from build123d import *

# Parameters (mm, degrees)
SKETCH1_R           = 2.1
BOSS_EXTRUDE1_DEPTH = 154
FILLET1_R           = 0.5


with BuildPart() as part:
    # Sketch1 → Boss-Extrude1 (new body)
    with BuildSketch(Plane.XY):
        Polygon((-20, -10), (-15.5, -10), (-15.1, -10), (-13.1, -8), (-15.5, -8), (-15.5, -6.560660172), (-12.539339828, -3.6), (-7.460660172, -3.6), (-4.5, -6.560660172), (-4.5, -8), (-6.9, -8), (-4.9, -10), (5.313777138, -10), (7.313777138, -8), (4.5, -8), (4.5, -6.560660172), (7.460660172, -3.6), (12.539339828, -3.6), (15.5, -6.560660172), (15.5, -8), (13.513777138, -8), (15.1, -10), (15.5, -10), (20, -10), (20, -5.5), (20, -5.1), (18, -3.1), (18, -5.5), (16.560660172, -5.5), (13.6, -2.539339828), (13.6, 2.539339828), (16.560660172, 5.5), (18, 5.5), (18, 3.1), (20, 5.1), (20, 5.5), (20, 10), (15.5, 10), (15.1, 10), (13.1, 8), (15.5, 8), (15.5, 6.560660172), (12.539339828, 3.6), (7.460660172, 3.6), (4.5, 6.560660172), (4.5, 8), (7.313777138, 8), (5.313777138, 10), (-4.9, 10), (-6.9, 8), (-4.5, 8), (-4.5, 6.560660172), (-7.460660172, 3.6), (-12.539339828, 3.6), (-15.5, 6.560660172), (-15.5, 8), (-13.1, 8), (-15.1, 10), (-15.5, 10), (-20, 10), (-20, 5.5), (-20, 5.1), (-18, 3.1), (-18, 5.5), (-16.560660172, 5.5), (-13.6, 2.539339828), (-13.6, -2.539339828), (-16.560660172, -5.5), (-18, -5.5), (-18, -3.1), (-20, -5.1), (-20, -5.5), align=None)
        with Locations((-10, 0)):
            Circle(SKETCH1_R, mode=Mode.SUBTRACT)
        with Locations((10, 0)):
            Circle(SKETCH1_R, mode=Mode.SUBTRACT)
        Polygon((3, -5.939339828), (3, -8), (-3, -8), (-3, -5.939339828), (-6.4, -2.539339828), (-6.4, 2.539339828), (-3, 5.939339828), (-3, 8), (3, 8), (3, 5.939339828), (6.4, 2.539339828), (6.4, -2.539339828), align=None, mode=Mode.SUBTRACT)
    extrude(amount=BOSS_EXTRUDE1_DEPTH)

    # Fillet1
    fillet1_edges = [part.edges().sort_by_distance(p)[0] for p in [
        (-20, 10, 77),
        (20, 10, 77),
        (20, -10, 77),
        (-20, -10, 77),
    ]]
    fillet(fillet1_edges, radius=FILLET1_R)


solid = part.part
CAD build for the part. Positions are in the model's coordinates, mm. A direction names the side the tool comes from. Round coordinates to 2 decimals unless told otherwise and drop trailing zeros. Order: outer loops, then holes, each group sorted by start corner. A loop starts at its lowest first (then second) coordinate and runs counter-clockwise, first axis right, second up. Notation, with made-up numbers: M 67.25,85.25 L 83.25,85.25 A23 ccw 83.25,101.25 Z; hole C 65,-22 d8. An arc over 180 degrees is marked long. Use one line per item in the form item = value.
Q1. Saw through at D-D on z = 13. State how many separate pieces and enclosed holes the cut face has, then the cut area to 3 significant figures.
Recorded:
separate_pieces = 1
enclosed_holes = 3
area = 283 mm^2
Q2. Saw through at B-B on y = 0. Give the cut face in (x, z), then the cut area to 3 significant figures.
Recorded:
outline = M -13.6,0 L -12.1,0 L -12.1,154 L -13.6,154 Z; M -7.9,0 L -6.4,0 L -6.4,154 L -7.9,154 Z; M 6.4,0 L 7.9,0 L 7.9,154 L 6.4,154 Z; M 12.1,0 L 13.6,0 L 13.6,154 L 12.1,154 Z
area = 924 mm^2
Q3. Which spindle directions (+Z, -Z, +X, -X, +Y, -Y) get a long thin tool onto all of the face, cutting with end or side? Do faces 1 (the flat face through (4.68, 4.26, 75.92)), 2 (the flat face through (4.4, -5.1, 0)). Say none if no direction does.
Recorded:
face_1 = +Z, -Z
face_2 = -Z, +X, -X, +Y, -Y
Q4. Two-plate mould, pull along X, no slides. Class faces 3 (the flat face through (-4.68, -4.26, 75.92)), 4 (the flat face through (5.96, -5.1, 75.92)), 5 (the flat face through (17, 10, 76)), 6 (the flat face through (-20, 7, 76)): +X half, -X half, draft (parallel to the pull), parting line (faces both ways), or undercut.
Recorded:
face_3 = undercut
face_4 = undercut
face_5 = draft
face_6 = -X half
Q5. Saw through at C-C on x = 9.5. Give the cut face in (y, z), then the cut area to 3 significant figures.
Recorded:
outline = M -3.6,0 L -2.04,0 L -2.04,154 L -3.6,154 Z; M 2.04,0 L 3.6,0 L 3.6,154 L 2.04,154 Z
area = 481 mm^2
Q6. Saw through at A-A on x = -10. Give the cut face in (y, z).
Recorded:
outline = M -3.6,0 L -2.1,0 L -2.1,154 L -3.6,154 Z; M 2.1,0 L 3.6,0 L 3.6,154 L 2.1,154 Z
Q7. Probe L1, parallel to Y at x = -10, z = 115; L2, parallel to X at y = -7.25, z = 89; L3, parallel to Y at x = 1, z = 55. List the from-to ranges inside material, lowest first.
Recorded:
L1 = -3.6 to -2.1, 2.1 to 3.6
L2 = -20 to -15.5, -4.5 to -3, 3 to 4.5, 15.5 to 20
L3 = -10 to -8, 8 to 10
Q8. Flat gauge pins, fed straight in: P1, Ø1.9, axis at x = -15, z = 70.5, coming from the -Y side; P2, Ø5.5, axis at y = 0.5, z = 112.5, coming from the -X side; P3, Ø4, axis at x = 10.5, z = 52, coming from the +Y side; P4, Ø4, axis at y = 0, z = 47.5, coming from the -X side. Where does each tip first touch, or does it go through?
Recorded:
P1 = -10
P2 = -18.15
P3 = 3.6
P4 = -13.6
